Verification items for the finished model (mm, model axes). A direction names the side the tool comes from. Coordinates: 2 decimals unless noted, no trailing zeros. Order: outer loops, then holes, each group sorted by start corner. A loop starts at its lowest first (then second) coordinate and runs counter-clockwise, first axis right, second up. Notation, with made-up numbers: M 1,17.25 L 34,17.25 A25 ccw 34,47.25 Z; hole C -39,-2.5 d5. An arc over 180 degrees is marked long. Answer as a JSON object with one key per item and string values. Group by question number.
(1) Gauge pin test, flat ends, axial feed: pin 1 Ø3 at (x, z) = (129.5, 2) entering from -Y; pin 2 Ø3 at (x, y) = (69, -14.5) entering from -Z; pin 3 Ø5 at (x, y) = (-12, 0) entering from -Z; pin 4 Ø1.5 at (y, z) = (0, 1) entering from +X. Record the tip position at first contact, or that the pin passes through.
(2) Cross-section at C-C (z = 2.5). Enter the section's corners in (x, y), plus the area to 3 significant figures.
(3) Cross-section at A-A (y = 0). Enter the section's corners in (x, z).
(4) Cross-section at B-B (x = 21.5). Enter the section's corners in (y, z).
(5) Mould release check, pull along X, two halves, no side actions. Record for faces 1 (the face through (7.474, 11.744, 4.93)), 2 (the face through (159.1, -19.14, 5.48)), 3 (the face through (77, -20, 5)): released by +X, released by -X, zero draft, split by the parting line, or undercut.
(6) Access from +Z, -Z, +X, -X, +Y, -Y to the whole of each face (thin tool, end or side, straight path). Record for faces 4 (the face through (77.4, -19.14, 1.9)), 5 (the face through (159.14, -0.24, 1.9)).
(7) Material ranges on line 1 (Y direction, x = 12, z = 5.75); line 2 (X direction, y = -0.5, z = 1.5); line 3 (X direction, y = 10.5, z = 1.5), recorded low to high.
from build123d import *

# Parameters (mm, degrees)
SKETCH8_R             = 20
BOSS_EXTRUDE6_DEPTH   = 10
BOSS_EXTRUDE7_START   = 1
BOSS_EXTRUDE7_DEPTH   = 9
F_4_0MM_DOWEL_HOLE2_D = 4
FILLET4_R             = 3


with BuildPart() as part:
    # Sketch8 → Boss-Extrude6 (new body)
    with BuildSketch(Plane.XY):
        Circle(SKETCH8_R)
    extrude(amount=BOSS_EXTRUDE6_DEPTH)

    # Sketch8<4> → Boss-Extrude7 (add)
    with BuildSketch(Plane.XY.offset(BOSS_EXTRUDE7_START)):
        with BuildLine():
            Line((160, 20), (0, 20))
            ThreePointArc((0, 20), (14.142135624, 14.142135624), (20, 0))
            ThreePointArc((20, 0), (14.142135624, -14.142135624), (0, -20))
            Line((0, -20), (160, -20))
            Line((160, -20), (160, 20))
        make_face()
    extrude(amount=BOSS_EXTRUDE7_DEPTH)

    # Ø4.0mm Dowel Hole2 (through all)
    with Locations(Plane.XY.offset(10)):
        with Locations((6, 10.392304845), (12, 0), (6, -10.392304845), (-6, -10.392304845), (-12, 0), (-6, 10.392304845)):
            Hole(F_4_0MM_DOWEL_HOLE2_D / 2)

    # Fillet4
    # the kernel refuses this fillet: 3 mm, written as the material it takes off along each edge
    with BuildSketch(Plane(origin=(157, 17, 4), x_dir=(1, 0, 0), z_dir=(0, 0, -1))) as fillet4_piece_1_section:
        Polygon((0, 0), (FILLET4_R, 0), (FILLET4_R, -FILLET4_R), (0, -FILLET4_R), align=None)
    fillet4_piece_1 = extrude(amount=FILLET4_R, mode=Mode.PRIVATE)
    fillet4_piece_1 = fillet4_piece_1 - Plane(origin=(157, 17, 4), x_dir=(-0.7071067811865475, -0.7071067811865475, 0), z_dir=(0, 0, -1)) * Sphere(FILLET4_R, mode=Mode.PRIVATE)
    add(fillet4_piece_1, mode=Mode.SUBTRACT)
    with BuildSketch(Plane(origin=(157, 17, 7), x_dir=(1, 0, 0), z_dir=(0, 0, 1))) as fillet4_piece_2_section:
        Polygon((0, 0), (FILLET4_R, 0), (FILLET4_R, FILLET4_R), (0, FILLET4_R), align=None)
    fillet4_piece_2 = extrude(amount=FILLET4_R, mode=Mode.PRIVATE)
    fillet4_piece_2 = fillet4_piece_2 - Plane(origin=(157, 17, 7), x_dir=(-0.7071067811865475, -0.7071067811865475, 0), z_dir=(0, 0, 1)) * Sphere(FILLET4_R, mode=Mode.PRIVATE)
    add(fillet4_piece_2, mode=Mode.SUBTRACT)
    with BuildSketch(Plane(origin=(157, -17, 4), x_dir=(0, -1, 0), z_dir=(0, 0, -1))) as fillet4_piece_3_section:
        Polygon((0, 0), (FILLET4_R, 0), (FILLET4_R, -FILLET4_R), (0, -FILLET4_R), align=None)
    fillet4_piece_3 = extrude(amount=FILLET4_R, mode=Mode.PRIVATE)
    fillet4_piece_3 = fillet4_piece_3 - Plane(origin=(157, -17, 4), x_dir=(-0.7071067811865475, 0.7071067811865475, 0), z_dir=(0, 0, -1)) * Sphere(FILLET4_R, mode=Mode.PRIVATE)
    add(fillet4_piece_3, mode=Mode.SUBTRACT)
    with BuildSketch(Plane(origin=(157, -17, 7), x_dir=(0, 0, 1), z_dir=(0, -1, 0))) as fillet4_piece_4_section:
        Polygon((0, 0), (FILLET4_R, 0), (FILLET4_R, -FILLET4_R), (0, -FILLET4_R), align=None)
    fillet4_piece_4 = extrude(amount=FILLET4_R, mode=Mode.PRIVATE)
    fillet4_piece_4 = fillet4_piece_4 - Plane(origin=(157, -17, 7), x_dir=(-0.7071067811865475, 0, -0.7071067811865475), z_dir=(0, -1, 0)) * Sphere(FILLET4_R, mode=Mode.PRIVATE)
    add(fillet4_piece_4, mode=Mode.SUBTRACT)
    with BuildSketch(Plane(origin=(160, 20, 4), x_dir=(-1, 0, 0), z_dir=(0, 0, 1))) as fillet4_piece_5:
        with BuildLine():
            CenterArc((FILLET4_R, FILLET4_R), FILLET4_R, 180, 90)
            Line((0, FILLET4_R), (0, 0))
            Line((0, 0), (FILLET4_R, 0))
        make_face()
    extrude(amount=3, mode=Mode.SUBTRACT)
    with BuildSketch(Plane(origin=(157, 20, 1), x_dir=(0, -1, 0), z_dir=(-1, 0, 0))) as fillet4_piece_6_section:
        with BuildLine():
            CenterArc((FILLET4_R, FILLET4_R), FILLET4_R, 180, 90)
            Line((0, FILLET4_R), (0, 0))
            Line((0, 0), (FILLET4_R, 0))
        make_face()
    fillet4_piece_6 = extrude(amount=164.5, mode=Mode.PRIVATE)
    fillet4_piece_6 = fillet4_piece_6 - Plane(origin=(0, 0, 1.692410686), x_dir=(1, 0, 0), z_dir=(0, 0, -1)) * Cylinder(20, 341, mode=Mode.PRIVATE)
    add(fillet4_piece_6, mode=Mode.SUBTRACT)
    with BuildSketch(Plane(origin=(160, -17, 1), x_dir=(-1, 0, 0), z_dir=(0, 1, 0))) as fillet4_piece_7:
        with BuildLine():
            CenterArc((FILLET4_R, FILLET4_R), FILLET4_R, 180, 90)
            Line((0, FILLET4_R), (0, 0))
            Line((0, 0), (FILLET4_R, 0))
        make_face()
    extrude(amount=34, mode=Mode.SUBTRACT)
    with BuildSketch(Plane(origin=(-7.5, -20, 1), x_dir=(0, 1, 0), z_dir=(1, 0, 0))) as fillet4_piece_8_section:
        with BuildLine():
            CenterArc((FILLET4_R, FILLET4_R), FILLET4_R, 180, 90)
            Line((0, FILLET4_R), (0, 0))
            Line((0, 0), (FILLET4_R, 0))
        make_face()
    fillet4_piece_8 = extrude(amount=164.5, mode=Mode.PRIVATE)
    fillet4_piece_8 = fillet4_piece_8 - Plane(origin=(0, 0, 1.692408431), x_dir=(1, 0, 0), z_dir=(0, 0, -1)) * Cylinder(20, 341, mode=Mode.PRIVATE)
    add(fillet4_piece_8, mode=Mode.SUBTRACT)
    with BuildSketch(Plane(origin=(0, 0, 10), x_dir=(0, 1, 0), z_dir=(1, 0, 0))) as fillet4_piece_9:
        with BuildLine():
            CenterArc((20 - FILLET4_R, -FILLET4_R), FILLET4_R, 0, 90)
            Line((20 - FILLET4_R, 0), (20, 0))
            Line((20, 0), (20, -FILLET4_R))
        make_face()
    revolve(axis=Axis((0, 0, 10), (0, 0, 1)), revolution_arc=180, mode=Mode.SUBTRACT)
    with BuildSketch(Plane(origin=(0, -20, 10), x_dir=(0, 0, -1), z_dir=(1, 0, 0))) as fillet4_piece_10:
        with BuildLine():
            CenterArc((FILLET4_R, FILLET4_R), FILLET4_R, 180, 90)
            Line((0, FILLET4_R), (0, 0))
            Line((0, 0), (FILLET4_R, 0))
        make_face()
    extrude(amount=157, mode=Mode.SUBTRACT)
    with BuildSketch(Plane(origin=(160, -17, 10), x_dir=(-1, 0, 0), z_dir=(0, 1, 0))) as fillet4_piece_11:
        with BuildLine():
            CenterArc((FILLET4_R, -FILLET4_R), FILLET4_R, 90, 90)
            Line((0, -FILLET4_R), (0, 0))
            Line((0, 0), (FILLET4_R, 0))
        make_face()
    extrude(amount=34, mode=Mode.SUBTRACT)
    with BuildSketch(Plane(origin=(160, -20, 4), x_dir=(-1, 0, 0), z_dir=(0, 0, 1))) as fillet4_piece_12:
        with BuildLine():
            CenterArc((FILLET4_R, -FILLET4_R), FILLET4_R, 90, 90)
            Line((0, -FILLET4_R), (0, 0))
            Line((0, 0), (FILLET4_R, 0))
        make_face()
    extrude(amount=3, mode=Mode.SUBTRACT)
    with BuildSketch(Plane(origin=(157, 20, 10), x_dir=(0, -1, 0), z_dir=(-1, 0, 0))) as fillet4_piece_13:
        with BuildLine():
            CenterArc((FILLET4_R, -FILLET4_R), FILLET4_R, 90, 90)
            Line((0, -FILLET4_R), (0, 0))
            Line((0, 0), (FILLET4_R, 0))
        make_face()
    extrude(amount=157, mode=Mode.SUBTRACT)


solid = part.part
Taken from the geometry:
{
 "1": {"pin 1": "stops at y = -19.96", "pin 2": "stops at z = 1", "pin 3": "stops at z = 0", "pin 4": "stops at x = 158.98"},
 "2": {"outline": "M 3.99,-19.6 L 157,-19.6 A2.6 ccw 159.6,-17 L 159.6,17 A2.6 ccw 157,19.6 L 3.99,19.6 A20 ccw long Z; hole C -12,0 d4; hole C -6,-10.39 d4; hole C -6,10.39 d4; hole C 6,-10.39 d4; hole C 6,10.39 d4; hole C 12,0 d4", "area": "6,810 mm²"},
 "3": {"outline": "M -20,0 L -14,0 L -14,10 L -17,10 A3 ccw -20,7 Z; M -10,0 L 10,0 L 10,10 L -10,10 Z; M 14,0 L 20,0 L 20,1 L 157,1 A3 ccw 160,4 L 160,7 A3 ccw 157,10 L 14,10 Z"},
 "4": {"outline": "M -20,4 A3 ccw -17,1 L 17,1 A3 ccw 20,4 L 20,7 A3 ccw 17,10 L -17,10 A3 ccw -20,7 Z"},
 "5": {"face 1": "undercut", "face 2": "released by +X", "face 3": "zero draft"},
 "6": {"face 4": "-Z, +X, -Y", "face 5": "-Z, +X, +Y, -Y"},
 "7": {"line 1": "y = -20 to -2, 2 to 20", "line 2": "x = -19.99 to -13.94, -10.06 to 10.06, 13.94 to 158.66", "line 3": "x = -17.02 to -8, -4 to 4, 8 to 158.66"}
}
